The model under review builds one solid part; all positions refer to its coordinate system, in mm. A direction names the side the tool comes from. Round coordinates to 2 decimals unless told otherwise and drop trailing zeros. Loops run counter-clockwise (first coordinate to the right, second up) from the corner with the lowest first, then second, coordinate; pieces in that order, holes last. Notation, with made-up numbers: (7.25, 60) - (26.25, 60) arc R38 cw to (26.25, 98) - close; hole circle Ø5 at (25, 57.25). An arc over 180 degrees is marked (long way). Answer as CSV lines item,"result".
from build123d import *

# Parameters (mm, degrees)
SKETCH_1_W          = 47
SKETCH_1_H          = 21.3
EXTRUDE_1_DEPTH     = 5
SKETCH_2_R          = 1.55
SKETCH_2_R_2        = 8.5
CUT_EXTRUDE_1_DEPTH = 13.95
SKETCH_7_W          = 47
SKETCH_7_H          = 20
EXTRUDE_3_DEPTH     = 3
SKETCH_3_W          = 12
SKETCH_3_H          = 2.5
CUT_EXTRUDE_2_DEPTH = 13.95
FILLET_4_R          = 0.5
SKETCH_11_R         = 2
CUT_EXTRUDE_4_DEPTH = 3
FILLET_5_R          = 0.5


with BuildPart() as part:
    # 草圖1 → 填料-伸長1 (new body)
    with BuildSketch(Plane.XY):
        Rectangle(SKETCH_1_W, SKETCH_1_H)
    extrude(amount=EXTRUDE_1_DEPTH)

    # 草圖2 → 除料-伸長1 (cut)
    with BuildSketch(Plane.XY.offset(5)):
        with Locations((-20.1, -8.15)):
            Circle(SKETCH_2_R)
        with Locations((20.5, 8.15)):
            Circle(SKETCH_2_R)
        with Locations((-12.5, 0)):
            Circle(SKETCH_2_R_2)
        with Locations((13, 0)):
            Circle(SKETCH_2_R_2)
    extrude(amount=-CUT_EXTRUDE_1_DEPTH, mode=Mode.SUBTRACT)

    # 草圖7 → 填料-伸長3 (add)
    with BuildSketch(Plane.XZ.offset(10.65)):
        with Locations((0, -5)):
            Rectangle(SKETCH_7_W, SKETCH_7_H)
    extrude(amount=EXTRUDE_3_DEPTH)

    # 草圖3 → 除料-伸長2 (cut)
    with BuildSketch(Plane.XY.offset(5)):
        with Locations((0.5, 9.4)):
            Rectangle(SKETCH_3_W, SKETCH_3_H)
    extrude(amount=-CUT_EXTRUDE_2_DEPTH, mode=Mode.SUBTRACT)

    # 圓角4
    fillet_4_edges = [part.edges().sort_by_distance(p)[0] for p in [
        (15, 10.65, 5),
        (6.5, 10.65, 2.5),
        (15, 10.65, 0),
        (-14.5, 10.65, 0),
        (-5.5, 10.65, 2.5),
        (-14.5, 10.65, 5),
        (-23.5, 10.65, 2.5),
        (-23.5, -1.5, 5),
        (-23.5, -13.65, -5),
        (-23.5, -12.15, -15),
        (-23.5, -10.65, -7.5),
        (-23.5, 0, 0),
        (23.5, -10.65, -7.5),
        (23.5, -12.15, -15),
        (23.5, -13.65, -5),
        (23.5, -1.5, 5),
        (23.5, 10.65, 2.5),
        (23.5, 0, 0),
    ]]
    fillet(fillet_4_edges, radius=FILLET_4_R)

    # 草圖11 → 除料-伸長4 (cut)
    with BuildSketch(Plane(origin=(0, -10.65, 0), x_dir=(1, 0, 0), z_dir=(0, 1, 0))):
        with Locations(Location((0, 10, 0), (0, 0, 270))):
            Circle(SKETCH_11_R)
        with Locations(Location((16, 10, 0), (0, 0, 270))):
            Circle(SKETCH_11_R)
        with Locations(Location((-16, 10, 0), (0, 0, 270))):
            Circle(SKETCH_11_R)
    extrude(amount=-CUT_EXTRUDE_4_DEPTH, mode=Mode.SUBTRACT)

    # 圓角5
    # the kernel refuses this fillet: 0.5 mm, written as the material it takes off along each edge
    with BuildSketch(Plane(origin=(-23, -13.15, -14.5), x_dir=(0, 0, -1), z_dir=(0, -1, 0))) as fillet_5_piece_1_section:
        Polygon((0, 0), (FILLET_5_R, 0), (FILLET_5_R, -FILLET_5_R), (0, -FILLET_5_R), align=None)
    fillet_5_piece_1 = extrude(amount=FILLET_5_R, mode=Mode.PRIVATE)
    fillet_5_piece_1 = fillet_5_piece_1 - Plane(origin=(-23, -13.15, -14.5), x_dir=(0.7071067811865475, 0, 0.7071067811865475), z_dir=(0, -1, 0)) * Sphere(FILLET_5_R, mode=Mode.PRIVATE)
    add(fillet_5_piece_1, mode=Mode.SUBTRACT)
    with BuildSketch(Plane(origin=(-23, -11.15, -14.5), x_dir=(0, 0, -1), z_dir=(0, 1, 0))) as fillet_5_piece_2_section:
        Polygon((0, 0), (FILLET_5_R, 0), (FILLET_5_R, FILLET_5_R), (0, FILLET_5_R), align=None)
    fillet_5_piece_2 = extrude(amount=FILLET_5_R, mode=Mode.PRIVATE)
    fillet_5_piece_2 = fillet_5_piece_2 - Plane(origin=(-23, -11.15, -14.5), x_dir=(0.7071067811865475, 0, 0.7071067811865475), z_dir=(0, 1, 0)) * Sphere(FILLET_5_R, mode=Mode.PRIVATE)
    add(fillet_5_piece_2, mode=Mode.SUBTRACT)
    with BuildSketch(Plane(origin=(23, -11.15, -14.5), x_dir=(0, 0, -1), z_dir=(0, 1, 0))) as fillet_5_piece_3_section:
        Polygon((0, 0), (FILLET_5_R, 0), (FILLET_5_R, -FILLET_5_R), (0, -FILLET_5_R), align=None)
    fillet_5_piece_3 = extrude(amount=FILLET_5_R, mode=Mode.PRIVATE)
    fillet_5_piece_3 = fillet_5_piece_3 - Plane(origin=(23, -11.15, -14.5), x_dir=(-0.7071067811865475, 0, 0.7071067811865475), z_dir=(0, 1, 0)) * Sphere(FILLET_5_R, mode=Mode.PRIVATE)
    add(fillet_5_piece_3, mode=Mode.SUBTRACT)
    with BuildSketch(Plane(origin=(23, -13.15, -14.5), x_dir=(0, 0, -1), z_dir=(0, -1, 0))) as fillet_5_piece_4_section:
        Polygon((0, 0), (FILLET_5_R, 0), (FILLET_5_R, FILLET_5_R), (0, FILLET_5_R), align=None)
    fillet_5_piece_4 = extrude(amount=FILLET_5_R, mode=Mode.PRIVATE)
    fillet_5_piece_4 = fillet_5_piece_4 - Plane(origin=(23, -13.15, -14.5), x_dir=(-0.7071067811865475, 0, 0.7071067811865475), z_dir=(0, -1, 0)) * Sphere(FILLET_5_R, mode=Mode.PRIVATE)
    add(fillet_5_piece_4, mode=Mode.SUBTRACT)
    with BuildSketch(Plane(origin=(-23, -13.65, -15), x_dir=(0, 0, 1), z_dir=(1, 0, 0))) as fillet_5_piece_5:
        with BuildLine():
            CenterArc((FILLET_5_R, -FILLET_5_R), FILLET_5_R, 90, 90)
            Line((0, -FILLET_5_R), (0, 0))
            Line((0, 0), (FILLET_5_R, 0))
        make_face()
    extrude(amount=46, mode=Mode.SUBTRACT)
    with BuildSketch(Plane(origin=(-23, -10.65, -15), x_dir=(0, 0, 1), z_dir=(1, 0, 0))) as fillet_5_piece_6:
        with BuildLine():
            CenterArc((FILLET_5_R, FILLET_5_R), FILLET_5_R, 180, 90)
            Line((0, FILLET_5_R), (0, 0))
            Line((0, 0), (FILLET_5_R, 0))
        make_face()
    extrude(amount=46, mode=Mode.SUBTRACT)


solid = part.part
1. Draft analysis for pull direction X (two halves, no side actions). For faces 4 (the face through (6.5, 9, 3)), 5 (the face through (23.5, -4, 1)), 6 (the face through (-15, 10.65, 2)), state which applies: +X half, -X half, draft (parallel to the pull), parting line (faces both ways), or undercut.
Numbers:
face 4,"undercut"
face 5,"+X half"
face 6,"draft"
2. Tool access review of faces 1 (the face through (-5.5, 9, 3)), 2 (the face through (18, -12, -10)), 3 (the face through (0, -10.65, -7)): name each direction out of +Z, -Z, +X, -X, +Y, -Y from which nothing blocks a thin tool from reaching the whole face with its end or side.
Numbers:
face 1,"+Z, -Z, +Y"
face 2,"+Y, -Y"
face 3,"-Z, +X, -X, +Y"
3. Take a section at C-C (x = 9). State the section outline as (y, z) points, plus the area to 3 significant figures.
Numbers:
outline,"(-13.65, -14.5) arc R0.5 ccw to (-13.15, -15) - (-11.15, -15) arc R0.5 ccw to (-10.65, -14.5) - (-10.65, 0) - (-7.5, 0) - (-7.5, 5) - (-13.65, 5) - close; (7.5, 0) - (10.15, 0) arc R0.5 ccw to (10.65, 0.5) - (10.65, 4.5) arc R0.5 ccw to (10.15, 5) - (7.5, 5) - close"
area,"91.3 mm²"
4. Take a section at D-D (z = -9.75). State the section outline as (x, y) points.
Numbers:
outline,"(-23.5, -13.15) arc R0.5 ccw to (-23, -13.65) - (-17.98, -13.65) - (-17.98, -10.65) - (-23, -10.65) arc R0.5 ccw to (-23.5, -11.15) - close; (-14.02, -13.65) - (-1.98, -13.65) - (-1.98, -10.65) - (-14.02, -10.65) - close; (1.98, -13.65) - (14.02, -13.65) - (14.02, -10.65) - (1.98, -10.65) - close; (17.98, -13.65) - (23, -13.65) arc R0.5 ccw to (23.5, -13.15) - (23.5, -11.15) arc R0.5 ccw to (23, -10.65) - (17.98, -10.65) - close"
5. Take a section at B-B (z = 2.75). State the section outline as (x, y) points, plus the area to 3 significant figures.
Numbers:
outline,"(-23.5, -13.15) arc R0.5 ccw to (-23, -13.65) - (23, -13.65) arc R0.5 ccw to (23.5, -13.15) - (23.5, 10.15) arc R0.5 ccw to (23, 10.65) - (7, 10.65) arc R0.5 ccw to (6.5, 10.15) - (6.5, 8.15) - (-5.5, 8.15) - (-5.5, 10.15) arc R0.5 ccw to (-6, 10.65) - (-23, 10.65) arc R0.5 ccw to (-23.5, 10.15) - close; hole circle Ø3.1 at (-20.1, -8.15); hole circle Ø17 at (-12.5, 0); hole circle Ø17 at (13, 0); hole circle Ø3.1 at (20.5, 8.15)"
area,"643 mm²"
6. Wall thickness on probe 1 along Y at (x, z) = (20.5, 2.1); probe 2 along Y at (x, z) = (13, 1.5); probe 3 along Y at (x, z) = (-20.1, 3.7): over which ranges is each line inside the solid? List them lowest first.
Numbers:
probe 1,"y = -13.65 to -4, 4 to 6.6, 9.7 to 10.65"
probe 2,"y = -13.65 to -8.5, 8.5 to 10.65"
probe 3,"y = -13.65 to -9.7, -6.6 to -3.81, 3.81 to 10.65"
7. Clearance check with flat-ended pins moving along their axes: pin 1 (10 mm diameter, centred on x = 11.5, y = -3.5, fed in from -Z); pin 2 (4 mm diameter, centred on x = -0.5, z = 2.5, fed in from +Y); pin 3 (5 mm diameter, centred on x = 16, z = -10, fed in from +Y). State where each tip first meets the part, or that it passes through.
Numbers:
pin 1,"stops at z = 0"
pin 2,"stops at y = 8.15"
pin 3,"stops at y = -10.65"
8. Take a section at A-A (x = 20.5). State the section outline as (y, z) points, plus the area to 3 significant figures.
Numbers:
outline,"(-13.65, -14.5) arc R0.5 ccw to (-13.15, -15) - (-11.15, -15) arc R0.5 ccw to (-10.65, -14.5) - (-10.65, 0) - (-4, 0) - (-4, 5) - (-13.65, 5) - close; (4, 0) - (6.6, 0) - (6.6, 5) - (4, 5) - close; (9.7, 0) - (10.15, 0) arc R0.5 ccw to (10.65, 0.5) - (10.65, 4.5) arc R0.5 ccw to (10.15, 5) - (9.7, 5) - close"
area,"111 mm²"
